```python
from build123d import *

# Parameters (mm, degrees)
SKETCH1_W                = 135.031416385
SKETCH1_H                = 114.879
SKETCH1_R                = 2.1
BOSS_EXTRUDE1_DEPTH      = 6.35
BOSS_EXTRUDE2_DEPTH      = 6.35
BOSS_EXTRUDE2_DEPTH_BACK = 6.35
SKETCH4_W                = 135.031416385
SKETCH4_H                = 6.35
BOSS_EXTRUDE3_DEPTH      = 6.35
FILLET2_R                = 2.54
FILLET3_R                = 2.54


with BuildPart() as part:
    # Sketch1 → Boss-Extrude1 (new body)
    with BuildSketch(Plane(origin=(0, 0, -64.874447619), x_dir=(-1, 0, 0), z_dir=(0, 0, -1))):
        with Locations((-131.653812741, -75.312789105)):
            Rectangle(SKETCH1_W, SKETCH1_H)
        with Locations((-179.484520933, -22.318289105)):
            Circle(SKETCH1_R, mode=Mode.SUBTRACT)
        with Locations((-78.138520933, -22.318289105)):
            Circle(SKETCH1_R, mode=Mode.SUBTRACT)
        with Locations((-78.138520933, -123.029289105)):
            Circle(SKETCH1_R, mode=Mode.SUBTRACT)
        with Locations((-179.484520933, -123.029289105)):
            Circle(SKETCH1_R, mode=Mode.SUBTRACT)
    extrude(amount=BOSS_EXTRUDE1_DEPTH)

    # Sketch4 → Boss-Extrude2 (add, two sides: drawn at the far end of the back side and taken through both)
    with BuildSketch(Plane(origin=(0, 0, -71.224447619), x_dir=(-1, 0, 0), z_dir=(0, 0, -1)).offset(-BOSS_EXTRUDE2_DEPTH_BACK)):
        with Locations((-131.653812741, -135.927289105)):
            Rectangle(SKETCH4_W, SKETCH4_H)
        with Locations((-131.653812741, -14.698289105)):
            Rectangle(SKETCH4_W, SKETCH4_H)
    extrude(amount=BOSS_EXTRUDE2_DEPTH + BOSS_EXTRUDE2_DEPTH_BACK)

    # Sketch5 → Boss-Extrude3 (add)
    with BuildSketch(Plane(origin=(0, 0, -77.574447619), x_dir=(-1, 0, 0), z_dir=(0, 0, -1))):
        with BuildLine():
            Line((-118.238104548, 4.476710895), (-118.238104548, -11.523289105))
            Line((-118.238104548, -11.523289105), (-102.238104548, -11.523289105))
            Line((-102.238104548, -11.523289105), (-102.238104548, -7.523289105))
            Line((-102.238104548, -7.523289105), (-110.364104548, -7.523289105))
            ThreePointArc((-110.364104548, -7.523289105), (-114.364104548, -3.523289105), (-110.364104548, 0.476710895))
            Line((-110.364104548, 0.476710895), (-102.238104548, 0.476710895))
            Line((-102.238104548, 0.476710895), (-102.238104548, 4.476710895))
            Line((-102.238104548, 4.476710895), (-118.238104548, 4.476710895))
        make_face()
        with BuildLine():
            Line((-169.23476894, -139.102289105), (-185.23476894, -139.102289105))
            Line((-185.23476894, -139.102289105), (-185.23476894, -155.102289105))
            Line((-185.23476894, -155.102289105), (-169.23476894, -155.102289105))
            Line((-169.23476894, -155.102289105), (-169.23476894, -151.102289105))
            Line((-169.23476894, -151.102289105), (-177.30996894, -151.102289105))
            ThreePointArc((-177.30996894, -151.102289105), (-181.30996894, -147.102289105), (-177.30996894, -143.102289105))
            Line((-177.30996894, -143.102289105), (-169.23476894, -143.102289105))
            Line((-169.23476894, -143.102289105), (-169.23476894, -139.102289105))
        make_face()
    extrude(amount=-BOSS_EXTRUDE3_DEPTH)

    # Fillet2
    fillet2_edges = [part.edges().sort_by_distance(p)[0] for p in [
        (118.238104548, 4.476710895, -74.399447619),
    ]]
    fillet(fillet2_edges, radius=FILLET2_R)

    # Fillet3
    fillet3_edges = [part.edges().sort_by_distance(p)[0] for p in [
        (185.23476894, -155.102289105, -74.399447619),
    ]]
    fillet(fillet3_edges, radius=FILLET3_R)


solid = part.part
```
Build history of the part. All positions in model axes, mm. A direction names the side the tool comes from. Give positions to 0.01 mm unless a question says otherwise; leave off trailing zeros. Loops run counter-clockwise (first coordinate to the right, second up) from the corner with the lowest first, then second, coordinate; pieces in that order, holes last.
1) Drop flat-ended pins along their axis: P1, Ø3.5, axis at x = 78.14, y = -22.32, coming from the -Z side; P2, Ø3, axis at y = -141.5, z = -73.5, coming from the -X side; P3, Ø5, axis at x = 167, z = -73.5, coming from the +Y side; P4, Ø5, axis at x = 113, z = -73, coming from the -Y side. Give the stop position or say it passes through.
Values follow:
P1: passes through
P2: stops at x = 169.23
P3: stops at y = -11.52
P4: stops at y = -139.1
2) Band-saw the part on C-C on x = 84. List the corners of the cut face in (y, z), then the cut area to 3 significant figures.
Values follow:
outline: (-139.1, -77.57) - (-132.75, -77.57) - (-132.75, -71.22) - (-17.87, -71.22) - (-17.87, -77.57) - (-11.52, -77.57) - (-11.52, -64.87) - (-139.1, -64.87) - close
area: 891 mm2
3) Band-saw the part on B-B on z = -74. List the corners of the cut face in (x, y).
Values follow:
outline: (64.14, -139.1) - (169.23, -139.1) - (169.23, -143.1) - (177.31, -143.1) arc R4 cw to (177.31, -151.1) - (169.23, -151.1) - (169.23, -155.1) - (182.69, -155.1) arc R2.54 ccw to (185.23, -152.56) - (185.23, -139.1) - (199.17, -139.1) - (199.17, -132.75) - (64.14, -132.75) - close; (64.14, -17.87) - (199.17, -17.87) - (199.17, -11.52) - (118.24, -11.52) - (118.24, 1.94) arc R2.54 ccw to (115.7, 4.48) - (102.24, 4.48) - (102.24, 0.48) - (110.36, 0.48) arc R4 cw to (110.36, -7.52) - (102.24, -7.52) - (102.24, -11.52) - (64.14, -11.52) - close
4) Band-saw the part on A-A on x = 174. List the corners of the cut face in (y, z).
Values follow:
outline: (-155.1, -77.57) - (-151.1, -77.57) - (-151.1, -71.22) - (-155.1, -71.22) - close; (-143.1, -77.57) - (-132.75, -77.57) - (-132.75, -71.22) - (-17.87, -71.22) - (-17.87, -77.57) - (-11.52, -77.57) - (-11.52, -64.87) - (-139.1, -64.87) - (-139.1, -71.22) - (-143.1, -71.22) - close
5) Probe line 1 along Y through (x, z) = (102.5, -71.75); line 2 along Y through (x, z) = (172, -71.5); line 3 along Y through (x, z) = (126, -76.75). List the from-to ranges inside material, lowest first.
Values follow:
line 1: y = -139.1 to -132.75, -17.87 to -7.52, 0.48 to 4.48
line 2: y = -155.1 to -151.1, -143.1 to -132.75, -17.87 to -11.52
line 3: y = -139.1 to -132.75, -17.87 to -11.52
6) Two-plate mould, pull along X, no slides. Class faces 1 (the face through (109, 4.477, -74)), 2 (the face through (78.59, -125.08, -68)), 3 (the face through (102.238, 2, -74)), 4 (the face through (185.235, -146, -74)): released by +X, released by -X, zero draft, split by the parting line, or undercut.
Values follow:
face 1: zero draft
face 2: undercut
face 3: released by -X
face 4: released by +X
7) Band-saw the part on D-D on y = -80. List the corners of the cut face in (x, z), then the cut area to 3 significant figures.
Values follow:
outline: (64.14, -71.22) - (199.17, -71.22) - (199.17, -64.87) - (64.14, -64.87) - close
area: 857 mm2
8) 3-axis set-ups, long thin cutter, end or side, ignore diameter. For faces 5 (the face through (181, -145, -71.224)), 6 (the face through (102.238, -10, -74)), 7 (the face through (106, 0.477, -74)): which of +Z, -Z, +X, -X, +Y, -Y reach the whole face in a straight line?
Values follow:
face 5: +Z, +X, -X, -Y
face 6: +Z, -Z, -X, +Y
face 7: +Z, -Z, -X
